```python
from build123d import *

# Parameters (mm, degrees)
SKETCH1_W           = 121
SKETCH1_H           = 50
BOSS_EXTRUDE1_DEPTH = 4
SKETCH2_W           = 4
SKETCH2_H           = 5
BOSS_EXTRUDE2_DEPTH = 4
LPATTERN1_COUNT     = 5
LPATTERN1_PITCH     = 10
SKETCH3_W           = 10
SKETCH3_H           = 4
BOSS_EXTRUDE3_DEPTH = 4
LPATTERN2_COUNT     = 3
LPATTERN2_PITCH     = 20
LPATTERN2_COL_COUNT = 3
LPATTERN2_COL_PITCH = 20
SKETCH4_W           = 10
SKETCH4_H           = 4
CUT_EXTRUDE1_DEPTH  = 135.688529578


with BuildPart() as part:
    # Sketch1 → Boss-Extrude1 (new body)
    with BuildSketch(Plane(origin=(0, 0, 0), x_dir=(1, 0, 0), z_dir=(0, 1, 0))):
        with Locations((60.5, -25)):
            Rectangle(SKETCH1_W, SKETCH1_H)
    extrude(amount=BOSS_EXTRUDE1_DEPTH)

    # Sketch2 → Boss-Extrude2 (add, through all)
    with BuildSketch(Plane(origin=(0, 0, 0), x_dir=(-1, 0, 0), z_dir=(0, -1, 0))):
        with Locations((2, -47.5)):
            Rectangle(SKETCH2_W, SKETCH2_H)
        with Locations((-123, -47.5)):
            Rectangle(SKETCH2_W, SKETCH2_H)
    boss_extrude2 = extrude(amount=-BOSS_EXTRUDE2_DEPTH)

    # LPattern1: Boss-Extrude2 ×5
    with Locations(*[(0, 0, -i * LPATTERN1_PITCH) for i in range(1, LPATTERN1_COUNT)]):
        add(boss_extrude2)

    # Sketch3 → Boss-Extrude3 (add, through all)
    with BuildSketch(Plane(origin=(0, 0, 0), x_dir=(-1, 0, 0), z_dir=(0, -1, 0))):
        with Locations((-60.5, 2)):
            Rectangle(SKETCH3_W, SKETCH3_H)
    boss_extrude3 = extrude(amount=-BOSS_EXTRUDE3_DEPTH)

    # LPattern2: Boss-Extrude3 ×3
    with Locations(*[(i * LPATTERN2_PITCH, 0, 0) for i in range(1, LPATTERN2_COUNT)]):
        add(boss_extrude3)

    # LPattern2 col: Boss-Extrude3 ×3
    with Locations(*[(-i * LPATTERN2_COL_PITCH, 0, 0) for i in range(1, LPATTERN2_COL_COUNT)]):
        add(boss_extrude3)

    # Sketch4 → Cut-Extrude1 (cut, through all)
    with BuildSketch(Plane.XZ):
        with Locations((20.5, 26)):
            Rectangle(SKETCH4_W, SKETCH4_H)
        with Locations((40.5, 26)):
            Rectangle(SKETCH4_W, SKETCH4_H)
        with Locations((60.5, 26)):
            Rectangle(SKETCH4_W, SKETCH4_H)
        with Locations((80.5, 26)):
            Rectangle(SKETCH4_W, SKETCH4_H)
        with Locations((100.5, 26)):
            Rectangle(SKETCH4_W, SKETCH4_H)
    extrude(amount=-CUT_EXTRUDE1_DEPTH, mode=Mode.SUBTRACT)


solid = part.part
```
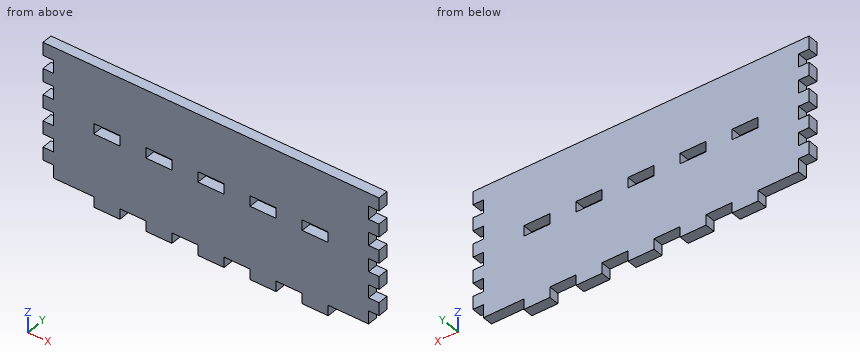
Source: CAD feature listing. Evaluate the final solid. Frame: model axes, mm. Coordinates: 2 decimals unless noted, no trailing zeros. Write each loop counter-clockwise with the first axis right and the second up, starting at its lowest first coordinate (ties: lowest second). Pieces come first, ordered by that corner, then holes. Notation, with made-up numbers: M 60,13 L 118,13 A31 ccw 118,37 Z; hole C 78.25,-39 d3. An arc over 180 degrees is marked long. Answer as a JSON object with one key per item and string values.
1. Ray query, L1, parallel to X at y = 3.55, z = -0.5; L2, parallel to X at y = 2.2, z = 27.5; L3, parallel to Z at x = 17, y = 3.05. Return the intervals inside material, ascending.
Evaluation:
{"L1": "15.5 to 25.5, 35.5 to 45.5, 55.5 to 65.5, 75.5 to 85.5, 95.5 to 105.5", "L2": "-4 to 15.5, 25.5 to 35.5, 45.5 to 55.5, 65.5 to 75.5, 85.5 to 95.5, 105.5 to 125", "L3": "-4 to 24, 28 to 50"}
2. Cut plane B-B on y = 1.15. State how many separate pieces and enclosed holes the cut face has, plus the area to 3 significant figures.
Evaluation:
{"separate pieces": "1", "enclosed holes": "5", "area": "6,250 mm^2"}
3. Contact query for flat-ended pins moving along their axis: P1, Ø1.2, axis at x = 92.5, y = 2.5, coming from the -Z side; P2, Ø1.2, axis at y = 3, z = -1.5, coming from the -X side; P3, Ø1.2, axis at y = 2.5, z = -1.5, coming from the +X side. Output: stop coordinate, or through.
Evaluation:
{"P1": "z = 0", "P2": "x = 15.5", "P3": "x = 105.5"}
4. Cut plane A-A on x = 78. Output: boundary loops of the cut face in (y, z).
Evaluation:
{"outline": "M 0,-4 L 4,-4 L 4,24 L 0,24 Z; M 0,28 L 4,28 L 4,50 L 0,50 Z"}
5. Cut plane C-C on z = 32.5. Output: boundary loops of the cut face in (x, y), plus the area to 3 significant figures.
Evaluation:
{"outline": "M 0,0 L 121,0 L 121,4 L 0,4 Z", "area": "484 mm^2"}
